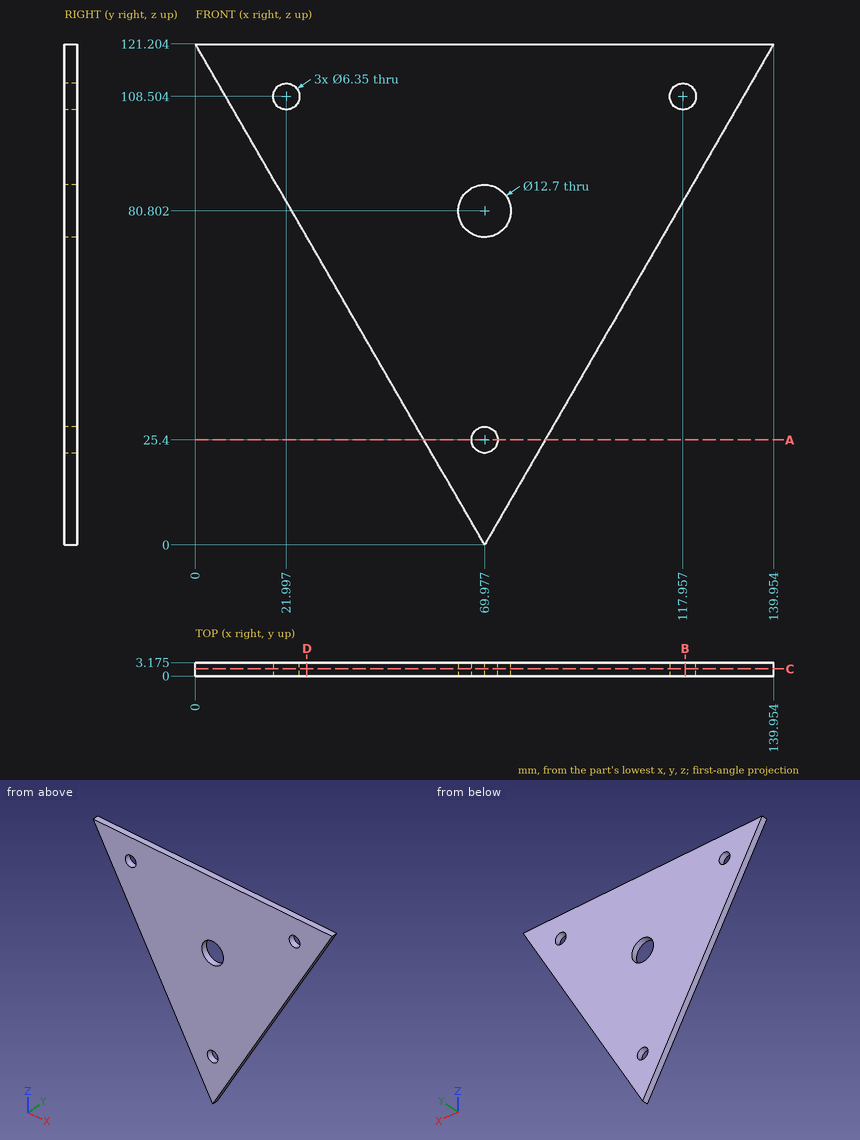
Verification items for this drawing (mm, ordinates from the low corner). Give positions to 0.01 mm unless a question says otherwise; leave off trailing zeros. Write each loop counter-clockwise with the first axis right and the second up, starting at its lowest first coordinate (ties: lowest second). Pieces come first, ordered by that corner, then holes. Notation, with made-up numbers: (40, 81) - (90, 81) arc R19 ccw to (90, 106) - close; hole circle Ø6 at (-40, 43). An arc over 180 degrees is marked (long way). Answer as CSV lines item,"result". Start each with the question number.
1. Depth check by flat-ended pin: pin 1 (1.5 mm diameter, centred on x = 41, y = 1, fed in from -Z); pin 2 (4 mm diameter, centred on x = 22, z = 108.5, fed in from -Y); pin 3 (1.5 mm diameter, centred on y = 2.5, z = 12, fed in from +X). Enter the tip coordinate at first touch or a pass-through.
2. Sectioned sample at A-A (z = 25.4). Record the boundary of the cut face in (x, y) (1 decimal).
3. Sectioned sample at B-B (x = 118.5). Record the boundary of the cut face in (y, z) (1 decimal).
4. Sectioned sample at C-C (y = 1.7). Count the separate pieces of the cut face and the enclosed holes in it, then the cut area to 3 significant figures.
5. Sectioned sample at D-D (x = 27). Record the boundary of the cut face in (y, z) (1 decimal).
6. Thickness scan on line 1 (X direction, y = 0.65, z = 109) (1 decimal); line 2 (Z direction, x = 119.5, y = 3) (1 decimal); line 3 (Z direction, x = 64.5, y = 1.2) (1 decimal). Record the ranges inside material, lowest first.
Derived:
1,pin 1,"z = 48.89"
1,pin 2,"through"
1,pin 3,"x = 77.34"
2,outline,"(55.3, 0) - (66.8, 0) - (66.8, 3.2) - (55.3, 3.2) - close; (73.2, 0) - (84.6, 0) - (84.6, 3.2) - (73.2, 3.2) - close"
3,outline,"(0, 84) - (3.2, 84) - (3.2, 105.4) - (0, 105.4) - close; (0, 111.6) - (3.2, 111.6) - (3.2, 121.2) - (0, 121.2) - close"
4,separate pieces,"1"
4,enclosed holes,"4"
4,area,"8,260 mm²"
5,outline,"(0, 74.4) - (3.2, 74.4) - (3.2, 121.2) - (0, 121.2) - close"
6,line 1,"7 to 18.9, 25.1 to 114.8, 121.1 to 132.9"
6,line 2,"85.8 to 105.7, 111.3 to 121.2"
6,line 3,"9.5 to 77.6, 84 to 121.2"
